Read the model definition and answer for the solid it produces. Units are mm, in the model's axes. Face numbers are marked on the shaded views. A direction names the side the tool comes from. Give positions to 0.01 mm unless a question says otherwise; leave off trailing zeros. Loops run counter-clockwise (first coordinate to the right, second up) from the corner with the lowest first, then second, coordinate; pieces in that order, holes last. Notation, with made-up numbers: (58.5, 72) - (65.5, 72) arc R28 cw to (65.5, 97) - close; hole circle Ø5 at (5, -7). An arc over 180 degrees is marked (long way). Write item = value, one per line.
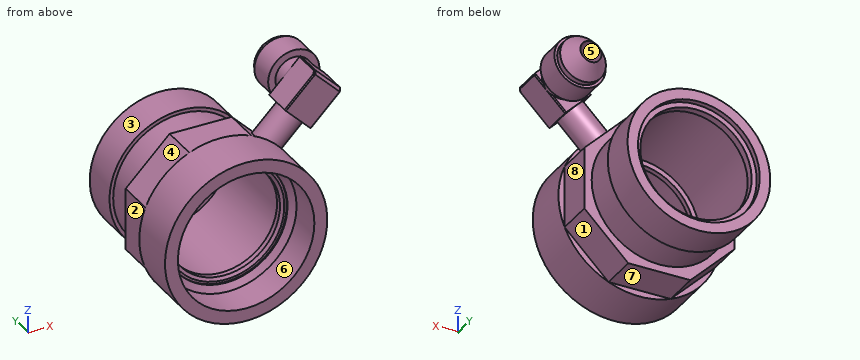
```python
from build123d import *

# Parameters (mm, degrees)
SKETCH_1_R                = 22
EXTRUDE_1_DEPTH           = 43
SKETCH_3_OUTSIDE_W        = 61.128
SKETCH_3_OUTSIDE_H        = 61.128
CUT_EXTRUDE_1_DEPTH       = 30
SKETCH_4_OUTSIDE_W        = 61.128
SKETCH_4_OUTSIDE_H        = 61.128
SKETCH_4_OUTSIDE_R        = 18.35
CUT_EXTRUDE_2_DEPTH       = 20
SKETCH_5_R                = 16.5
CUT_EXTRUDE_3_DEPTH       = 1.5
SKETCH_6_R                = 15.1
CUT_EXTRUDE_4_DEPTH       = 54.075418039
SKETCH_7_R                = 16.5
CUT_EXTRUDE_5_DEPTH       = 27
SKETCH_8_R                = 16.65
CUT_EXTRUDE_6_DEPTH       = 10.5
M39X2_02_D                = 37
M39X2_02_DEPTH            = 9
M39X2_02_TIP              = 11.115921452
SKETCH_14_R               = 3.95
EXTRUDE_2_DEPTH           = 9.6
SKETCH_15_W               = 10
SKETCH_15_H               = 8.5
EXTRUDE_3_DEPTH           = 12
CHAMFER_1_SIZE            = 0.8
CHAMFER_2_SIZE            = 0.3
SKETCH_18_R               = 5
EXTRUDE_4_DEPTH           = 3
CHAMFER_3_SIZE            = 0.3
SKETCH_19_R               = 6.95
EXTRUDE_5_DEPTH           = 7
SKETCH_21_R               = 6.2
EXTRUDE_6_DEPTH           = 1.5
SKETCH_24_R               = 2.85
CUT_EXTRUDE_7_DEPTH       = 22.5
CUT_EXTRUDE_11_REACH      = 69.044
CUT_EXTRUDE_11_END_RADIUS = 2.85
SKETCH_25_R               = 2.85
CUT_EXTRUDE_12_REACH      = 69.044
SKETCH_26_R               = 2.85
SKETCH_27_W               = 1
SKETCH_27_H               = 10


with BuildPart() as part:
    # Эскиз1 → Бобышка-Вытянуть1 (new body)
    with BuildSketch(Plane(origin=(0, 0, 0), x_dir=(1, 0, 0), z_dir=(0, 1, 0))):
        with Locations(Location((0, 0, 0), (0, 0, 270))):
            Circle(SKETCH_1_R)
    extrude(amount=EXTRUDE_1_DEPTH)

    # Эскиз3 outside → Вырез-Вытянуть1 (cut)
    with BuildSketch(Plane(origin=(0, 43, 0), x_dir=(1, 0, 0), z_dir=(0, 1, 0))):
        Rectangle(SKETCH_3_OUTSIDE_W, SKETCH_3_OUTSIDE_H)
        Polygon((20.325349715, -8.419035512), (20.325349715, 8.419035512), (8.419035512, 20.325349715), (-8.419035512, 20.325349715), (-20.325349715, 8.419035512), (-20.325349715, -8.419035512), (-8.419035512, -20.325349715), (8.419035512, -20.325349715), align=None, mode=Mode.SUBTRACT)
    extrude(amount=-CUT_EXTRUDE_1_DEPTH, mode=Mode.SUBTRACT)

    # Эскиз4 outside → Вырез-Вытянуть2 (cut)
    with BuildSketch(Plane(origin=(0, 43, 0), x_dir=(1, 0, 0), z_dir=(0, 1, 0))):
        Rectangle(SKETCH_4_OUTSIDE_W, SKETCH_4_OUTSIDE_H)
        with Locations(Location((0, 0, 0), (0, 0, 270))):
            Circle(SKETCH_4_OUTSIDE_R, mode=Mode.SUBTRACT)
    extrude(amount=-CUT_EXTRUDE_2_DEPTH, mode=Mode.SUBTRACT)

    # Эскиз5 → Вырез-Вытянуть3 (cut)
    with BuildSketch(Plane(origin=(0, 43, 0), x_dir=(1, 0, 0), z_dir=(0, 1, 0))):
        with Locations(Location((0, 0, 0), (0, 0, 270))):
            Circle(SKETCH_5_R)
    extrude(amount=-CUT_EXTRUDE_3_DEPTH, mode=Mode.SUBTRACT)

    # Эскиз6 → Вырез-Вытянуть4 (cut, through all)
    with BuildSketch(Plane(origin=(0, 43, 0), x_dir=(1, 0, 0), z_dir=(0, 1, 0))):
        with Locations(Location((0, 0, 0), (0, 0, 270))):
            Circle(SKETCH_6_R)
    extrude(amount=-CUT_EXTRUDE_4_DEPTH, mode=Mode.SUBTRACT)

    # Эскиз7 → Вырез-Вытянуть5 (cut)
    with BuildSketch(Plane(origin=(0, 39.5, 0), x_dir=(1, 0, 0), z_dir=(0, 1, 0))):
        with Locations(Location((0, 0, 0), (0, 0, 270))):
            Circle(SKETCH_7_R)
    extrude(amount=-CUT_EXTRUDE_5_DEPTH, mode=Mode.SUBTRACT)

    # Эскиз8 → Вырез-Вытянуть6 (cut)
    with BuildSketch(Plane.XZ):
        with Locations(Location((0, 0, 0), (0, 0, 270))):
            Circle(SKETCH_8_R)
    extrude(amount=-CUT_EXTRUDE_6_DEPTH, mode=Mode.SUBTRACT)

    # Отверстие обработанное метчиком M39x2.02
    with Locations(Plane(origin=(0, 0, 0), x_dir=(-1, 0, 0), z_dir=(0, -1, 0))):
        with Locations((0, 0)):
            Hole(M39X2_02_D / 2, depth=M39X2_02_DEPTH)
            with Locations((0, 0, -(M39X2_02_DEPTH + M39X2_02_TIP / 2))):  # 118° drill point
                Cone(0, M39X2_02_D / 2, M39X2_02_TIP, mode=Mode.SUBTRACT)

    # Эскиз14 → Бобышка-Вытянуть2 (add)
    with BuildSketch(Plane(origin=(14.372192614, 0, 14.372192614), x_dir=(0.7071067811865475, 0, -0.7071067811865476), z_dir=(0.7071067811865476, 0, 0.7071067811865475))):
        with Locations((0, 17.35)):
            Circle(SKETCH_14_R)
    extrude(amount=EXTRUDE_2_DEPTH)

    # Эскиз15 → Бобышка-Вытянуть3 (add)
    with BuildSketch(Plane(origin=(21.160417713, 0, 21.160417713), x_dir=(0.7071067811865475, 0, -0.7071067811865476), z_dir=(0.7071067811865476, 0, 0.7071067811865475))):
        with Locations((0, 17.35)):
            Rectangle(SKETCH_15_W, SKETCH_15_H)
    extrude(amount=EXTRUDE_3_DEPTH)

    # Фаска1
    chamfer_1_edges = [part.edges().sort_by_distance(p)[0] for p in [
        (29.645699087, 13.1, 29.645699087),
    ]]
    chamfer(chamfer_1_edges, length=CHAMFER_1_SIZE)

    # Фаска2
    chamfer_2_edges = [part.edges().sort_by_distance(p)[0] for p in [
        (26.110165181, 17.75, 33.181232993),
        (33.181232993, 17.75, 26.110165181),
        (28.655749594, 13.1, 21.584681782),
        (32.898390281, 13.5, 25.827322469),
        (21.584681782, 13.1, 28.655749594),
        (25.827322469, 13.5, 32.898390281),
    ]]
    chamfer(chamfer_2_edges, length=CHAMFER_2_SIZE)

    # Эскиз18 → Бобышка-Вытянуть4 (add)
    with BuildSketch(Plane(origin=(0, 21.6, 0), x_dir=(1, 0, 0), z_dir=(0, 1, 0))):
        with Locations(Location((26.110165181, -26.110165181, 0), (0, 0, 45))):
            Circle(SKETCH_18_R)
    extrude(amount=EXTRUDE_4_DEPTH)

    # Фаска3
    # the kernel refuses this chamfer: 0.3 mm, written as the material it takes off along each edge
    with BuildSketch(Plane(origin=(24.150415275, 21.6, 17.079347463), x_dir=(0.01944252080601493, -0.9996219169112965, -0.019442520806014937), z_dir=(0.7071067811865476, 0, 0.7071067811865475))) as chamfer_3_piece_1_section:
        Polygon((CHAMFER_3_SIZE * 0.999621916911, -CHAMFER_3_SIZE * 0.0274958766106), (-CHAMFER_3_SIZE * 0.0274958766106, -CHAMFER_3_SIZE * 0.999621916911), (0, 0), align=None)
    chamfer_3_piece_1 = extrude(amount=7.771504896, mode=Mode.PRIVATE)
    chamfer_3_piece_1 = chamfer_3_piece_1 - Plane(origin=(26.110165181, 21.497863029, 26.110165181), x_dir=(0.7071067811865476, 0, -0.7071067811865475), z_dir=(0, -1, 0)) * Cylinder(5, 17, mode=Mode.PRIVATE)
    add(chamfer_3_piece_1, mode=Mode.SUBTRACT)
    with BuildSketch(Plane(origin=(29.645699087, 21.6, 22.574631275), x_dir=(0.01944252080600918, -0.999621916911297, -0.019442520806009188), z_dir=(0.7071067811865476, 0, 0.7071067811865475))) as chamfer_3_piece_2_section:
        Polygon((CHAMFER_3_SIZE * 0.999621916911, -CHAMFER_3_SIZE * 0.0274958766106), (-CHAMFER_3_SIZE * 0.0274958766106, -CHAMFER_3_SIZE * 0.999621916911), (0, 0), align=None)
    chamfer_3_piece_2 = extrude(amount=5.471504896, mode=Mode.PRIVATE)
    chamfer_3_piece_2 = chamfer_3_piece_2 - Plane(origin=(26.110165181, 21.497295997, 26.110165181), x_dir=(0.7071067811865476, 0, -0.7071067811865475), z_dir=(0, -1, 0)) * Cylinder(5, 13, mode=Mode.PRIVATE)
    add(chamfer_3_piece_2, mode=Mode.SUBTRACT)
    with BuildSketch(Plane(origin=(17.079347463, 21.6, 24.150415275), x_dir=(-0.01944252080601493, -0.9996219169112965, 0.019442520806014937), z_dir=(0.7071067811865476, 0, 0.7071067811865475))) as chamfer_3_piece_3_section:
        Polygon((CHAMFER_3_SIZE * 0.999621916911, CHAMFER_3_SIZE * 0.0274958766106), (-CHAMFER_3_SIZE * 0.0274958766106, CHAMFER_3_SIZE * 0.999621916911), (0, 0), align=None)
    chamfer_3_piece_3 = extrude(amount=7.771504896, mode=Mode.PRIVATE)
    chamfer_3_piece_3 = chamfer_3_piece_3 - Plane(origin=(26.110165181, 21.497863029, 26.110165181), x_dir=(0.7071067811865476, 0, -0.7071067811865475), z_dir=(0, -1, 0)) * Cylinder(5, 17, mode=Mode.PRIVATE)
    add(chamfer_3_piece_3, mode=Mode.SUBTRACT)
    with BuildSketch(Plane(origin=(22.574631275, 21.6, 29.645699087), x_dir=(-0.01944252080602069, -0.9996219169112965, 0.01944252080602069), z_dir=(0.7071067811865476, 0, 0.7071067811865475))) as chamfer_3_piece_4_section:
        Polygon((CHAMFER_3_SIZE * 0.999621916911, CHAMFER_3_SIZE * 0.0274958766106), (-CHAMFER_3_SIZE * 0.0274958766106, CHAMFER_3_SIZE * 0.999621916911), (0, 0), align=None)
    chamfer_3_piece_4 = extrude(amount=5.471504896, mode=Mode.PRIVATE)
    chamfer_3_piece_4 = chamfer_3_piece_4 - Plane(origin=(26.110165181, 21.497295996, 26.110165181), x_dir=(0.7071067811865476, 0, -0.7071067811865475), z_dir=(0, -1, 0)) * Cylinder(5, 13, mode=Mode.PRIVATE)
    add(chamfer_3_piece_4, mode=Mode.SUBTRACT)

    # Эскиз19 → Бобышка-Вытянуть5 (add)
    with BuildSketch(Plane(origin=(0, 24.6, 0), x_dir=(1, 0, 0), z_dir=(0, 1, 0))):
        with Locations(Location((26.110165181, -26.110165181, 0), (0, 0, 270))):
            Circle(SKETCH_19_R)
    extrude(amount=EXTRUDE_5_DEPTH)

    # Эскиз21 → Бобышка-Вытянуть6 (add)
    with BuildSketch(Plane(origin=(0, 31.6, 0), x_dir=(1, 0, 0), z_dir=(0, 1, 0))):
        with Locations(Location((26.110165181, -26.110165181, 0), (0, 0, 270))):
            Circle(SKETCH_21_R)
    extrude(amount=EXTRUDE_6_DEPTH)

    # Эскиз22 → Повернуть1 (revolve)
    with BuildSketch(Plane(origin=(0, 0, 0), x_dir=(0.7071067811865477, 0, 0.7071067811865475), z_dir=(-0.7071067811865475, 0, 0.7071067811865477)), mode=Mode.PRIVATE) as revolve_1_sk:
        Polygon((36.925349715, 33.1), (36.925349715, 37.1), (39.775349715, 37.1), (43.125349715, 33.1), align=None)
    revolve(revolve_1_sk.sketch.rotate(Axis((26.110165181, -966.9, 26.110165181), (0, 1, 0)), 109.948443589), axis=Axis((26.110165181, -966.9, 26.110165181), (0, 1, 0)))

    # Эскиз24 → Вырез-Вытянуть7 (cut)
    with BuildSketch(Plane(origin=(0, 37.1, 0), x_dir=(1, 0, 0), z_dir=(0, 1, 0))):
        with Locations(Location((26.110165181, -26.110165181, 0), (0, 0, 270))):
            Circle(SKETCH_24_R)
    extrude(amount=-CUT_EXTRUDE_7_DEPTH, mode=Mode.SUBTRACT)

    # Вырез-Вытянуть11: up to this cylinder (the profile starts outside it)
    cut_extrude_11_end = Plane(origin=(26.110165181, 17.35, 26.110165181), z_dir=(0, 1, 0)) * Cylinder(CUT_EXTRUDE_11_END_RADIUS, 144.788, mode=Mode.PRIVATE)
    # Эскиз25 → Вырез-Вытянуть11 (cut, up to the surface)
    with BuildSketch(Plane(origin=(14.372192614, 0, 14.372192614), x_dir=(0.7071067811865475, 0, -0.7071067811865476), z_dir=(0.7071067811865476, 0, 0.7071067811865475)), mode=Mode.PRIVATE) as cut_extrude_11_sk1:
        with Locations((0, 17.35)):
            Circle(SKETCH_25_R)
    cut_extrude_11_tool1 = extrude(cut_extrude_11_sk1.sketch, amount=CUT_EXTRUDE_11_REACH, mode=Mode.PRIVATE) - cut_extrude_11_end
    add(cut_extrude_11_tool1.solids().sort_by_distance((14.372193, 17.35, 14.372193))[0], mode=Mode.SUBTRACT)

    # Эскиз26 → Вырез-Вытянуть12 (cut, up to next)
    with BuildSketch(Plane(origin=(14.372192614, 0, 14.372192614), x_dir=(0.7071067811865475, 0, -0.7071067811865476), z_dir=(0.7071067811865476, 0, 0.7071067811865475)), mode=Mode.PRIVATE) as cut_extrude_12_sk1:
        with Locations((0, 17.35)):
            Circle(SKETCH_26_R)
    cut_extrude_12_tool1 = extrude(cut_extrude_12_sk1.sketch, amount=-CUT_EXTRUDE_12_REACH, mode=Mode.PRIVATE) & part.part
    add(cut_extrude_12_tool1.solids().sort_by_distance((14.372193, 17.35, 14.372193))[0], mode=Mode.SUBTRACT)

    # Эскиз27 → Повернуть2 (revolve)
    with BuildSketch(Plane(origin=(0, 0, 0), x_dir=(0.7071067811865477, 0, 0.7071067811865475), z_dir=(-0.7071067811865475, 0, 0.7071067811865477)), mode=Mode.PRIVATE) as revolve_2_sk:
        with Locations((18.85, 38)):
            Rectangle(SKETCH_27_W, SKETCH_27_H)
    revolve(revolve_2_sk.sketch.rotate(Axis((0, 12.5, 0), (0, 1, 0)), 135), axis=Axis((0, 12.5, 0), (0, 1, 0)))


solid = part.part
```
1) A tool of negligible diameter and unlimited length cuts with its end or side. For the marked faces 1, 2, 3 and 4, from which of +Z, -Z, +X, -X, +Y, -Y can it reach the whole face along a straight path? Write none if from no direction.
Output:
face_1 = -Z, +X, +Y
face_2 = +Z, -Z, -X, +Y
face_3 = +Y
face_4 = +Z, -X, +Y
2) Find the intervals of material crossed by probe 1 along Z at (x, y) = (0, 6.5); probe 2 along Y at (x, z) = (19.5, -2.5); probe 3 along X at (y, z) = (2, 5.5), in increasing order.
Output:
probe_1 = -22 to -18.5, 18.5 to 22
probe_2 = 0 to 23
probe_3 = -21.3 to -17.66, 17.66 to 21.3
3) Each of these flat-tipped pins is pushed along its axis until it touches: P1, Ø0.8, axis at x = -21, z = 4, coming from the +Y side; P2, Ø5, axis at x = 18, y = 28, coming from the +Z side; P3, Ø7, axis at x = 27.5, z = 26, coming from the +Y side. Where does it stop, or does it pass through?
Output:
P1 = 13
P2 = 30.21
P3 = 37.1
4) The mould has two halves that part along X. Classify the marked faces 5, 6, 7 and 8: pulls with the +X half, pulls with the -X half, needs draft (parallel to the pull), parting line crosses it, or undercut.
Output:
face_5 = undercut
face_6 = undercut
face_7 = needs draft
face_8 = pulls with the +X half
5) A cutting plane is placed at A-A on y = 30. Determine the outline of the cut face in (x, z), then the cut area to 3 significant figures.
Output:
outline = circle Ø36.7 at (0, 0); circle Ø13.9 at (26.11, 26.11); hole circle Ø33 at (0, 0); hole circle Ø5.7 at (26.11, 26.11)
area = 329 mm²
6) A cutting plane is placed at B-B on y = 16. Determine the outline of the cut face in (x, z), then the cut area to 3 significant figures.
Output:
outline = (-20.33, -8.42) - (-8.42, -20.33) - (8.42, -20.33) - (20.33, -8.42) - (20.33, 8.42) - (17, 11.75) - (23.79, 18.54) - (24.7, 17.62) - (32.97, 25.9) - (32.97, 26.32) - (26.32, 32.97) - (25.9, 32.97) - (17.62, 24.7) - (18.54, 23.79) - (11.75, 17) - (8.42, 20.33) - (-8.42, 20.33) - (-20.33, 8.42) - close; hole (9.76, 13.31) arc R16.5 ccw (long way) to (13.31, 9.76) - (26.93, 23.38) arc R2.85 ccw (long way) to (23.38, 26.93) - close
area = 589 mm²
